CAD build for the part. Positions are in the model's coordinates, mm. A direction names the side the tool comes from. Round coordinates to 2 decimals unless told otherwise and drop trailing zeros. Loops run counter-clockwise (first coordinate to the right, second up) from the corner with the lowest first, then second, coordinate; pieces in that order, holes last.
```python
from build123d import *

# Parameters (mm, degrees)
SKETCH1_W            = 124.4
SKETCH1_H            = 111.7
BOSS_EXTRUDE1_DEPTH  = 2
SKETCH2_W            = 2
SKETCH2_H            = 101.7
BOSS_EXTRUDE2_DEPTH  = 38.5
SKETCH3_W            = 121.7
SKETCH3_H            = 4.7
BOSS_EXTRUDE3_DEPTH  = 3
SKETCH5_W            = 116.3
SKETCH5_H            = 2.7
CUT_EXTRUDE8_DEPTH   = 3
SKETCH14_W           = 121.7
SKETCH14_H           = 4.7
BOSS_EXTRUDE6_DEPTH  = 3
SKETCH15_W           = 116.3
SKETCH15_H           = 2.7
CUT_EXTRUDE14_DEPTH  = 3
SKETCH18_W           = 2
SKETCH18_H           = 0.3
BOSS_EXTRUDE7_DEPTH  = 35.2
SKETCH19_W           = 5.7
SKETCH19_H           = 4.7
BOSS_EXTRUDE8_DEPTH  = 32.2
SKETCH20_W           = 2.7
SKETCH20_H           = 32.2
CUT_EXTRUDE15_DEPTH  = 3
SKETCH21_W           = 2.7
SKETCH21_H           = 32.2
CUT_EXTRUDE16_DEPTH  = 3
SKETCH24_W           = 2.7
SKETCH24_H           = 32.2
CUT_EXTRUDE18_DEPTH  = 3
SKETCH25_W           = 2.7
SKETCH25_H           = 32.2
CUT_EXTRUDE19_DEPTH  = 3
SKETCH30_W           = 31
SKETCH30_H           = 14
SKETCH30_W_2         = 8
SKETCH30_H_2         = 7
CUT_EXTRUDE23_DEPTH  = 2
SKETCH31_W           = 6
SKETCH31_H           = 36.2
BOSS_EXTRUDE9_DEPTH  = 1.35
FILLET1_R            = 2
SKETCH33_W           = 99.7
SKETCH33_H           = 3
BOSS_EXTRUDE11_DEPTH = 1.35
SKETCH43_W           = 1.229805297
SKETCH43_H           = 112.077966817
CUT_EXTRUDE25_DEPTH  = 38.2
SKETCH47_W           = 57.12
SKETCH47_H           = 30
BOSS_EXTRUDE22_DEPTH = 38
SKETCH49_W           = 51.12
SKETCH49_H           = 30
CUT_EXTRUDE30_DEPTH  = 38
SKETCH51_W           = 2.352063359
SKETCH51_H           = 112.382279656
CUT_EXTRUDE33_DEPTH  = 77.2
SKETCH54_W           = 10
SKETCH54_H           = 4.16571725
SKETCH54_H_2         = 4.016594053
BOSS_EXTRUDE23_DEPTH = 9
SKETCH55_W           = 10
SKETCH55_H           = 3.950767522
SKETCH55_W_2         = 9.95127899
SKETCH55_H_2         = 4
BOSS_EXTRUDE24_DEPTH = 9
SKETCH56_R           = 1.1
CUT_EXTRUDE34_DEPTH  = 10
SKETCH57_R           = 1
CUT_EXTRUDE35_DEPTH  = 99.41
SKETCH58_W           = 30
SKETCH58_H           = 3
BOSS_EXTRUDE25_DEPTH = 43
SKETCH59_W           = 30
SKETCH59_H           = 3.021561104
BOSS_EXTRUDE26_DEPTH = 43
BOSS_EXTRUDE28_DEPTH = 6
BOSS_EXTRUDE29_DEPTH = 6
BOSS_EXTRUDE30_DEPTH = 6
BOSS_EXTRUDE31_DEPTH = 6
SKETCH64_W           = 30
SKETCH64_H           = 6.546083461
CUT_EXTRUDE36_DEPTH  = 101.12
SKETCH65_R           = 1.5
CUT_EXTRUDE37_DEPTH  = 6
SKETCH67_R           = 1.5
CUT_EXTRUDE39_DEPTH  = 6
SKETCH68_W           = 12.888719924
SKETCH68_H           = 13
BOSS_EXTRUDE32_DEPTH = 2
SKETCH69_W           = 13
SKETCH69_H           = 12.803280229
BOSS_EXTRUDE33_DEPTH = 2
SKETCH70_R           = 1.5
CUT_EXTRUDE40_DEPTH  = 10
SKETCH71_R           = 1.5
CUT_EXTRUDE41_DEPTH  = 10
SKETCH72_R           = 3.5
CUT_EXTRUDE42_DEPTH  = 2.2
SKETCH73_R           = 3.5
CUT_EXTRUDE43_DEPTH  = 2.2


with BuildPart() as part:
    # Sketch1 → Boss-Extrude1 (new body)
    with BuildSketch(Plane(origin=(0, 0, 0), x_dir=(1, 0, 0), z_dir=(0, 1, 0))):
        with Locations((62.2, 55.85)):
            Rectangle(SKETCH1_W, SKETCH1_H)
    extrude(amount=BOSS_EXTRUDE1_DEPTH)

    # Sketch2 → Boss-Extrude2 (add)
    with BuildSketch(Plane(origin=(0, 2, 0), x_dir=(1, 0, 0), z_dir=(0, 1, 0))):
        with Locations((122.05, 55.85)):
            Rectangle(SKETCH2_W, SKETCH2_H)
        with Locations((2.35, 55.85)):
            Rectangle(SKETCH2_W, SKETCH2_H)
    extrude(amount=BOSS_EXTRUDE2_DEPTH)

    # Sketch3 → Boss-Extrude3 (add)
    with BuildSketch(Plane(origin=(0, 2, 0), x_dir=(1, 0, 0), z_dir=(0, 1, 0))):
        with Locations((62.2, 2.35)):
            Rectangle(SKETCH3_W, SKETCH3_H)
    extrude(amount=BOSS_EXTRUDE3_DEPTH)

    # Sketch5 → Cut-Extrude8 (cut)
    with BuildSketch(Plane(origin=(0, 5, 0), x_dir=(1, 0, 0), z_dir=(0, 1, 0))):
        with Locations((62.2, 2.35)):
            Rectangle(SKETCH5_W, SKETCH5_H)
    extrude(amount=-CUT_EXTRUDE8_DEPTH, mode=Mode.SUBTRACT)

    # Sketch14 → Boss-Extrude6 (add)
    with BuildSketch(Plane(origin=(0, 2, 0), x_dir=(1, 0, 0), z_dir=(0, 1, 0))):
        with Locations((62.2, 109.35)):
            Rectangle(SKETCH14_W, SKETCH14_H)
    extrude(amount=BOSS_EXTRUDE6_DEPTH)

    # Sketch15 → Cut-Extrude14 (cut)
    with BuildSketch(Plane(origin=(0, 5, 0), x_dir=(1, 0, 0), z_dir=(0, 1, 0))):
        with Locations((62.2, 109.35)):
            Rectangle(SKETCH15_W, SKETCH15_H)
    extrude(amount=-CUT_EXTRUDE14_DEPTH, mode=Mode.SUBTRACT)

    # Sketch18 → Boss-Extrude7 (add)
    with BuildSketch(Plane(origin=(0, 2, 0), x_dir=(1, 0, 0), z_dir=(0, 1, 0))):
        with Locations((2.35, 106.85)):
            Rectangle(SKETCH18_W, SKETCH18_H)
        with Locations((122.05, 106.85)):
            Rectangle(SKETCH18_W, SKETCH18_H)
        with Locations((122.05, 4.85)):
            Rectangle(SKETCH18_W, SKETCH18_H)
        with Locations((2.35, 4.85)):
            Rectangle(SKETCH18_W, SKETCH18_H)
    extrude(amount=BOSS_EXTRUDE7_DEPTH)

    # Sketch19 → Boss-Extrude8 (add)
    with BuildSketch(Plane(origin=(0, 5, 0), x_dir=(1, 0, 0), z_dir=(0, 1, 0))):
        with Locations((120.2, 2.35)):
            Rectangle(SKETCH19_W, SKETCH19_H)
        with Locations((4.2, 2.35)):
            Rectangle(SKETCH19_W, SKETCH19_H)
        with Locations((120.2, 109.35)):
            Rectangle(SKETCH19_W, SKETCH19_H)
        with Locations((4.2, 109.35)):
            Rectangle(SKETCH19_W, SKETCH19_H)
    extrude(amount=BOSS_EXTRUDE8_DEPTH)

    # Sketch20 → Cut-Extrude15 (cut)
    with BuildSketch(Plane.ZY.offset(-117.35)):
        with Locations((-109.35, 21.1)):
            Rectangle(SKETCH20_W, SKETCH20_H)
    extrude(amount=-CUT_EXTRUDE15_DEPTH, mode=Mode.SUBTRACT)

    # Sketch21 → Cut-Extrude16 (cut)
    with BuildSketch(Plane(origin=(7.05, 0, 0), x_dir=(0, 0, -1), z_dir=(1, 0, 0))):
        with Locations((109.35, 21.1)):
            Rectangle(SKETCH21_W, SKETCH21_H)
    extrude(amount=-CUT_EXTRUDE16_DEPTH, mode=Mode.SUBTRACT)

    # Sketch24 → Cut-Extrude18 (cut)
    with BuildSketch(Plane(origin=(7.05, 0, 0), x_dir=(0, 0, -1), z_dir=(1, 0, 0))):
        with Locations((2.35, 21.1)):
            Rectangle(SKETCH24_W, SKETCH24_H)
    extrude(amount=-CUT_EXTRUDE18_DEPTH, mode=Mode.SUBTRACT)

    # Sketch25 → Cut-Extrude19 (cut)
    with BuildSketch(Plane.ZY.offset(-117.35)):
        with Locations((-2.35, 21.1)):
            Rectangle(SKETCH25_W, SKETCH25_H)
    extrude(amount=-CUT_EXTRUDE19_DEPTH, mode=Mode.SUBTRACT)

    # Sketch30 → Cut-Extrude23 (cut)
    with BuildSketch(Plane.ZY.offset(-1.35)):
        with Locations((-28.5, 33.5)):
            Rectangle(SKETCH30_W, SKETCH30_H)
        with Locations((-82.2, 37)):
            Rectangle(SKETCH30_W_2, SKETCH30_H_2)
    extrude(amount=-CUT_EXTRUDE23_DEPTH, mode=Mode.SUBTRACT)

    # Sketch31 → Boss-Extrude9 (add)
    with BuildSketch(Plane(origin=(123.05, 0, 0), x_dir=(0, 0, -1), z_dir=(1, 0, 0))):
        with Locations((3, 20.1)):
            Rectangle(SKETCH31_W, SKETCH31_H)
        with Locations((108.7, 20.1)):
            Rectangle(SKETCH31_W, SKETCH31_H)
    extrude(amount=BOSS_EXTRUDE9_DEPTH)

    # Fillet1
    fillet1_edges = [part.edges().sort_by_distance(p)[0] for p in [
        (0, 1, 0),
        (124.4, 19.1, 0),
        (124.4, 19.1, -111.7),
        (0, 1, -111.7),
    ]]
    fillet(fillet1_edges, radius=FILLET1_R)

    # Sketch33 → Boss-Extrude11 (add)
    with BuildSketch(Plane(origin=(123.05, 0, 0), x_dir=(0, 0, -1), z_dir=(1, 0, 0))):
        with Locations((55.85, 3.5)):
            Rectangle(SKETCH33_W, SKETCH33_H)
    extrude(amount=BOSS_EXTRUDE11_DEPTH)

    # Sketch43 → Cut-Extrude25 (cut, through all)
    with BuildSketch(Plane(origin=(0, 37.2, 0), x_dir=(1, 0, 0), z_dir=(0, 1, 0))):
        with Locations((0.614902649, 56.193231497)):
            Rectangle(SKETCH43_W, SKETCH43_H)
    extrude(amount=-CUT_EXTRUDE25_DEPTH, mode=Mode.SUBTRACT)

    # Sketch47 → Boss-Extrude22 (add)
    with BuildSketch(Plane(origin=(0, 0, 0), x_dir=(-1, 0, 0), z_dir=(0, -1, 0))):
        with Locations((-62.2, 55.85)):
            Rectangle(SKETCH47_W, SKETCH47_H)
    extrude(amount=BOSS_EXTRUDE22_DEPTH)

    # Sketch49 → Cut-Extrude30 (cut)
    with BuildSketch(Plane(origin=(0, -38, 0), x_dir=(-1, 0, 0), z_dir=(0, -1, 0))):
        with Locations((-62.2, 55.85)):
            Rectangle(SKETCH49_W, SKETCH49_H)
    extrude(amount=-CUT_EXTRUDE30_DEPTH, mode=Mode.SUBTRACT)

    # Sketch51 → Cut-Extrude33 (cut, through all)
    with BuildSketch(Plane(origin=(0, 38.2, 0), x_dir=(1, 0, 0), z_dir=(0, 1, 0))):
        with Locations((124.22603168, 56.299711796)):
            Rectangle(SKETCH51_W, SKETCH51_H)
    extrude(amount=-CUT_EXTRUDE33_DEPTH, mode=Mode.SUBTRACT)

    # Sketch54 → Boss-Extrude23 (add)
    with BuildSketch(Plane.ZY.offset(-1.35)):
        with Locations((-5, 35.117141375)):
            Rectangle(SKETCH54_W, SKETCH54_H)
        with Locations((-106.7, 35.191702973)):
            Rectangle(SKETCH54_W, SKETCH54_H_2)
    extrude(amount=BOSS_EXTRUDE23_DEPTH)

    # Sketch55 → Boss-Extrude24 (add)
    with BuildSketch(Plane(origin=(123.05, 0, 0), x_dir=(0, 0, -1), z_dir=(1, 0, 0))):
        with Locations((5, 35.224616239)):
            Rectangle(SKETCH55_W, SKETCH55_H)
        with Locations((106.724360505, 35.2)):
            Rectangle(SKETCH55_W_2, SKETCH55_H_2)
    extrude(amount=BOSS_EXTRUDE24_DEPTH)

    # Sketch56 → Cut-Extrude34 (cut)
    with BuildSketch(Plane(origin=(0, 37.2, 0), x_dir=(1, 0, 0), z_dir=(0, 1, 0))):
        with Locations((-3.1, 106.7)):
            Circle(SKETCH56_R)
        with Locations((127.5, 106.7)):
            Circle(SKETCH56_R)
        with Locations((127.5, 5)):
            Circle(SKETCH56_R)
        with Locations((-3.1, 5)):
            Circle(SKETCH56_R)
    extrude(amount=-CUT_EXTRUDE34_DEPTH, mode=Mode.SUBTRACT)

    # Sketch57 → Cut-Extrude35 (cut, through all)
    with BuildSketch(Plane(origin=(90.76, 0, 0), x_dir=(0, 0, -1), z_dir=(1, 0, 0))):
        with Locations((45.85, -34)):
            Circle(SKETCH57_R)
        with Locations((65.85, -34)):
            Circle(SKETCH57_R)
    extrude(amount=-CUT_EXTRUDE35_DEPTH, mode=Mode.SUBTRACT)

    # Sketch58 → Boss-Extrude25 (add)
    with BuildSketch(Plane(origin=(90.76, 0, 0), x_dir=(0, 0, -1), z_dir=(1, 0, 0))):
        with Locations((55.85, -29.25)):
            Rectangle(SKETCH58_W, SKETCH58_H)
    extrude(amount=BOSS_EXTRUDE25_DEPTH)

    # Sketch59 → Boss-Extrude26 (add)
    with BuildSketch(Plane.ZY.offset(-33.64)):
        with Locations((-55.85, -29.239219448)):
            Rectangle(SKETCH59_W, SKETCH59_H)
    extrude(amount=BOSS_EXTRUDE26_DEPTH)

    # Sketch61 → Boss-Extrude28 (add)
    with BuildSketch(Plane.XY.offset(-40.85)):
        Polygon((90.76, -21.75), (96.76, -27.75), (90.76, -27.75), align=None)
    extrude(amount=-BOSS_EXTRUDE28_DEPTH)

    # Sketch62 → Boss-Extrude29 (add)
    with BuildSketch(Plane(origin=(0, 0, -70.85), x_dir=(-1, 0, 0), z_dir=(0, 0, -1))):
        Polygon((-90.76, -21.75), (-90.76, -27.75), (-96.76, -27.75), align=None)
    extrude(amount=-BOSS_EXTRUDE29_DEPTH)

    # Sketch60 → Boss-Extrude30 (add)
    with BuildSketch(Plane.XY.offset(-40.85)):
        Polygon((27.64, -27.728438896), (33.64, -21.728438896), (33.64, -27.728438896), align=None)
    extrude(amount=-BOSS_EXTRUDE30_DEPTH)

    # Sketch63 → Boss-Extrude31 (add)
    with BuildSketch(Plane(origin=(0, 0, -70.85), x_dir=(-1, 0, 0), z_dir=(0, 0, -1))):
        Polygon((-33.64, -22.069435851), (-33.64, -27.728438896), (-27.64, -27.728438896), align=None)
    extrude(amount=-BOSS_EXTRUDE31_DEPTH)

    # Sketch64 → Cut-Extrude36 (cut, through all)
    with BuildSketch(Plane.ZY.offset(-33.64)):
        with Locations((-55.85, -36.27304173)):
            Rectangle(SKETCH64_W, SKETCH64_H)
    extrude(amount=-CUT_EXTRUDE36_DEPTH, mode=Mode.SUBTRACT)

    # Sketch65 → Cut-Extrude37 (cut)
    with BuildSketch(Plane(origin=(0, -30.75, 0), x_dir=(-1, 0, 0), z_dir=(0, -1, 0))):
        with Locations((-125.11, 55.85)):
            Circle(SKETCH65_R)
    extrude(amount=-CUT_EXTRUDE37_DEPTH, mode=Mode.SUBTRACT)

    # Sketch67 → Cut-Extrude39 (cut)
    with BuildSketch(Plane.XZ.offset(30.75)):
        with Locations((-0.71, -55.85)):
            Circle(SKETCH67_R)
    extrude(amount=-CUT_EXTRUDE39_DEPTH, mode=Mode.SUBTRACT)

    # Sketch68 → Boss-Extrude32 (add)
    with BuildSketch(Plane(origin=(0, -27.728438896, 0), x_dir=(1, 0, 0), z_dir=(0, 1, 0))):
        with Locations((-0.765640038, 55.85)):
            Rectangle(SKETCH68_W, SKETCH68_H)
    extrude(amount=BOSS_EXTRUDE32_DEPTH)

    # Sketch69 → Boss-Extrude33 (add)
    with BuildSketch(Plane(origin=(0, -27.75, 0), x_dir=(1, 0, 0), z_dir=(0, 1, 0))):
        with Locations((125.11, 55.751640115)):
            Rectangle(SKETCH69_W, SKETCH69_H)
    extrude(amount=BOSS_EXTRUDE33_DEPTH)

    # Sketch70 → Cut-Extrude40 (cut)
    with BuildSketch(Plane(origin=(0, -30.75, 0), x_dir=(-1, 0, 0), z_dir=(0, -1, 0))):
        with Locations((-125.11, 55.85)):
            Circle(SKETCH70_R)
    extrude(amount=-CUT_EXTRUDE40_DEPTH, mode=Mode.SUBTRACT)

    # Sketch71 → Cut-Extrude41 (cut)
    with BuildSketch(Plane(origin=(0, -30.75, 0), x_dir=(-1, 0, 0), z_dir=(0, -1, 0))):
        with Locations((0.71, 55.85)):
            Circle(SKETCH71_R)
    extrude(amount=-CUT_EXTRUDE41_DEPTH, mode=Mode.SUBTRACT)

    # Sketch72 → Cut-Extrude42 (cut)
    with BuildSketch(Plane(origin=(0, -30.75, 0), x_dir=(-1, 0, 0), z_dir=(0, -1, 0))):
        with Locations((0.71, 55.85)):
            Circle(SKETCH72_R)
    extrude(amount=-CUT_EXTRUDE42_DEPTH, mode=Mode.SUBTRACT)

    # Sketch73 → Cut-Extrude43 (cut)
    with BuildSketch(Plane(origin=(0, -30.75, 0), x_dir=(-1, 0, 0), z_dir=(0, -1, 0))):
        with Locations((-125.11, 55.85)):
            Circle(SKETCH73_R)
    extrude(amount=-CUT_EXTRUDE43_DEPTH, mode=Mode.SUBTRACT)


solid = part.part
```
Item 1: Cut at C-C, the plane y = -12.5. Give the cut face in (x, z), plus the area to 3 significant figures.
Answers follow:
outline: (33.64, -70.85) - (36.64, -70.85) - (36.64, -40.85) - (33.64, -40.85) - close; (87.76, -70.85) - (90.76, -70.85) - (90.76, -40.85) - (87.76, -40.85) - close
area: 180 mm2
Item 2: Two-plate mould, pull along Z, no slides. Class faces 1 (the flat face through (121.05, 21, -55)), 2 (the flat face through (132.05, 35, -107)), 3 (the flat face through (61.9, 4.7, -111.7)), 4 (the flat face through (58, 4, -4.7)): released by +Z, released by -Z, zero draft, split by the parting line, or undercut.
Answers follow:
face 1: undercut
face 2: zero draft
face 3: released by -Z
face 4: undercut
Item 3: Cut at A-A, the plane x = 21.5. Give the cut face in (y, z), plus the area to 3 significant figures.
Answers follow:
outline: (-30.75, -70.85) - (-27.73, -70.85) - (-27.73, -40.85) - (-30.75, -40.85) - close; (0, -111.7) - (5, -111.7) - (5, -110.7) - (2, -110.7) - (2, -108) - (5, -108) - (5, -107) - (2, -107) - (2, -4.7) - (5, -4.7) - (5, -3.7) - (2, -3.7) - (2, -1) - (5, -1) - (5, 0) - (0, 0) - close
area: 326 mm2
Item 4: Cut at B-B, the plane z = -84.5. Give the cut face in (x, y).
Answers follow:
outline: (1.23, 0) - (123.05, 0) - (123.05, 40.5) - (121.05, 40.5) - (121.05, 2) - (3.35, 2) - (3.35, 33.5) - (1.35, 33.5) - (1.35, 2) - (1.23, 2) - close
Item 5: Probe line 1 (X direction, y = -26.6, z = -55.85); line 2 (Z direction, x = 127.5, y = 34.25); line 3 (X direction, y = -29.9, z = -55.85). List the from-to ranges inside material, lowest first.
Answers follow:
line 1: x = -7.21 to -2.21, 0.79 to 5.68, 33.64 to 36.64, 87.76 to 90.76, 118.61 to 123.61, 126.61 to 131.61
line 2: z = -111.7 to -107.8, -105.6 to -101.75, -10 to -6.1, -3.9 to 0
line 3: x = -9.36 to -4.21, 2.79 to 36.64, 87.76 to 121.61, 128.61 to 133.76
Item 6: Cut at D-D, the plane x = 47.5. Give the cut face in (y, z), plus the area to 3 significant figures.
Answers follow:
outline: (0, -111.7) - (5, -111.7) - (5, -110.7) - (2, -110.7) - (2, -108) - (5, -108) - (5, -107) - (2, -107) - (2, -4.7) - (5, -4.7) - (5, -3.7) - (2, -3.7) - (2, -1) - (5, -1) - (5, 0) - (0, 0) - close
area: 235 mm2
Item 7: 3-axis set-ups, long thin cutter, end or side, ignore diameter. For faces 5 (the cylindrical face through (127.69, -29.665, -58.215)), 6 (the flat face through (92, -26, -64.85)), 7 (the flat face through (62, 4, -3.7)), 8 (the flat face through (12, -27.728, -56)), 9 (the flat face through (30.6, -24.77, -43.81)): which of +Z, -Z, +X, -X, +Y, -Y reach the whole face in a straight line?
Answers follow:
face 5: -Y
face 6: +X
face 7: +Y
face 8: none
face 9: +Z, -Z, -X
Item 8: Flat gauge pins, fed straight in: P1, Ø1.1, axis at y = 22, z = -111, coming from the +X side; P2, Ø22, axis at y = -15, z = -57, coming from the +X side; P3, Ø1, axis at x = 113, z = -100.5, coming from the +Y side. Where does each tip first touch, or does it go through?
Answers follow:
P1: stops at x = 123.05
P2: stops at x = 131.61
P3: stops at y = 2
